The listing builds one solid part. Answer for the finished solid, in the listing's coordinates (mm). A direction names the side the tool comes from. Coordinates: 2 decimals unless noted, no trailing zeros. Order: outer loops, then holes, each group sorted by start corner. A loop starts at its lowest first (then second) coordinate and runs counter-clockwise, first axis right, second up.
Autodesk Inventor part; units mm, degrees
ref_plane "YZ Plane" through (0, 0, 0) normal (1, 0, 0) x (0, 1, 0)
ref_plane "XZ Plane" through (0, 0, 0) normal (0, 1, 0) x (-1, 0, 0)
ref_plane "XY Plane" through (0, 0, 0) normal (0, 0, 1) x (1, 0, 0)
sketch "Esboço1" plane through (0, 0, 0) normal (1, 0, 0) x (0, 1, 0)
  arc A0 (1, -4.9038) -> (-1, -4.9038) centre (0, 0) ccw
  line L0 (-1, -14.7248) -> (-1, -4.9038)
  line L1 (1, -14.72) -> (1, -4.9038)
  line L2 (1, -14.72) -> (5, -14.72)
  line L3 (5, -14.72) -> (5, -16.72)
  line L4 (5, -16.72) -> (-5, -16.72)
  line L5 (-1, -14.7248) -> (-4.9983, -14.7248)
  line L6 (-5, -16.72) -> (-7.74, -15.72)
  line L7 (-4.9983, -14.7248) -> (-7.74, -15.72)
extrude "Extrusão1" add sketch "Esboço1" along normal blind 4
sketch "Esboço2" plane through (4, 0, 0) normal (1, 0, 0) x (0, 0, -1)
  circle A0 centre (0, 0) radius 2.5
  dimension "d20" = 5
extrude "Extrusão2" add sketch "Esboço2" along normal blind 3
chamfer "Chanfro1" distance 0.5 angle 45 1 edges at (7, 0, 2.5) measured on face at (7, -0.6619, -1.2612)
(1) Find section B-B (y = 0). Write down the section's boundary in (x, z), and give its area (3 significant figures).
(2) Consider line 1 (X direction, y = 0.5, z = -14.25); line 2 (Y direction, x = 3.5, z = -8.5); line 3 (Z direction, x = 2, y = -4.25). Determine where each line is inside the solid, lowest interval first.
(3) Find section D-D (y = -4.75). Write down the section's boundary in (x, z).
(4) The mould has two halves that part along Z. Classify faces 4 (the face through (5.23, 2.44, 0.54)), 5 (the face through (2, 5, -16)), 6 (the face through (2, -0.2, 5)): released by +Z, released by -Z, zero draft, split by the parting line, or undercut.
(5) Find section C-C (z = 0). Write down the section's boundary in (x, y).
(6) For faces 1 (the face through (0, 0, -3)), 2 (the face through (2, -1, -10)), 3 (the face through (2, 1, -10)), determine the directions among +Z, -Z, +X, -X, +Y, -Y from which every point of the face is accessible in a straight line to the end or side of a thin tool.
(7) Each of these flat-tipped pins is pushed along its axis until it touches: pin 1 Ø1.5 at (y, z) = (-6, -2) entering from -X; pin 2 Ø1.2 at (x, z) = (1.5, -10.5) entering from -Y; pin 3 Ø2 at (x, z) = (3, -16) entering from +Y; pin 4 Ø2 at (x, z) = (2.5, -12.5) entering from +Y. Where does it stop, or does it pass through?
(8) Find section A-A (x = 3.25). Write down the section's boundary in (y, z), and give its area (3 significant figures).
Findings below:
1. outline: (0, -16.72) - (4, -16.72) - (4, -2.5) - (6.5, -2.5) - (7, -2) - (7, 2) - (6.5, 2.5) - (4, 2.5) - (4, 5) - (0, 5) - close
1. area: 102 mm2
2. line 1: x = 0 to 4
2. line 2: y = -1 to 1
2. line 3: z = -16.72 to -14.72, -2.64 to 2.64
3. outline: (0, -16.72) - (4, -16.72) - (4, -14.72) - (0, -14.72) - close; (0, -1.58) - (4, -1.58) - (4, 1.58) - (0, 1.58) - close
4. face 4: split by the parting line
4. face 5: zero draft
4. face 6: undercut
5. outline: (0, -5) - (4, -5) - (4, -2.5) - (6.5, -2.5) - (7, -2) - (7, 2) - (6.5, 2.5) - (4, 2.5) - (4, 5) - (0, 5) - close
6. face 1: +Z, -Z, -X, +Y, -Y
6. face 2: +X, -X, -Y
6. face 3: +X, -X, +Y
7. pin 1: passes through
7. pin 2: stops at y = -1
7. pin 3: stops at y = 5
7. pin 4: stops at y = 1
8. outline: (-7.74, -15.72) - (-5, -16.72) - (5, -16.72) - (5, -14.72) - (1, -14.72) - (1, -4.9) arc R5 ccw (long way) to (-1, -4.9) - (-1, -14.72) - (-5, -14.72) - close
8. area: 121 mm2
